from build123d import *

# Parameters (mm, degrees)
EXTRUDE_1_DEPTH = 30


with BuildPart() as part:
    # 草图1 → 拉伸-薄壁1 (new body)
    with BuildSketch(Plane(origin=(0, 0, 0), x_dir=(1, 0, 0), z_dir=(0, 1, 0))):
        Polygon((-10, -10), (70, -10), (70, 20), (49.5, 20), (49.5, 27), (26.5, 27), (26.5, 50), (20, 50), (20, 70), (-10, 70), align=None)
        Polygon((0, 0), (60, 0), (60, 10), (39.5, 10), (39.5, 17), (16.5, 17), (16.5, 40), (10, 40), (10, 60), (0, 60), align=None, mode=Mode.SUBTRACT)
    extrude(amount=EXTRUDE_1_DEPTH)


solid = part.part
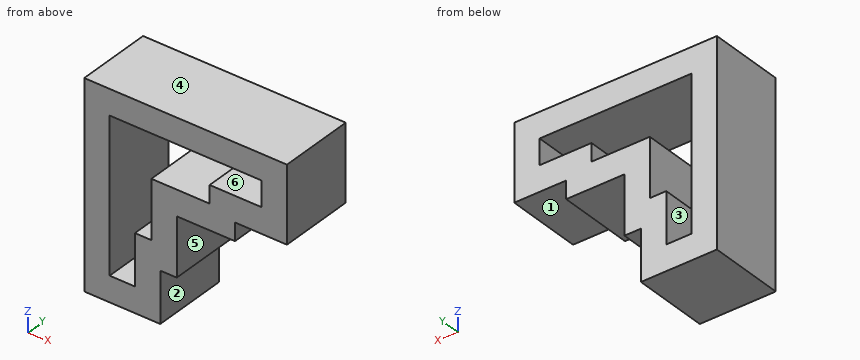
Input: part model. Units: mm. Frame: model coordinates. Face numbers are marked on the shaded views. A direction names the side the tool comes from. Give positions to 0.01 mm unless a question says otherwise; leave off trailing zeros. Order: outer loops, then holes, each group sorted by start corner. A loop starts at its lowest first (then second) coordinate and runs counter-clockwise, first axis right, second up.
Q1. Section A-A on x = 42. Output: boundary loops of the cut face in (y, z), and give its area (3 significant figures).
Checked values:
outline: (0, -27) - (30, -27) - (30, -10) - (0, -10) - close; (0, 0) - (30, 0) - (30, 10) - (0, 10) - close
area: 810 mm2
Q2. Contact query for flat-ended pins moving along their axis: pin 1 Ø10 at (y, z) = (19.5, -60) entering from +X; pin 2 Ø9 at (x, y) = (26.5, 16.5) entering from -Z; pin 3 Ø6 at (x, z) = (25, -24.5) entering from -Y; pin 4 Ø16.5 at (x, y) = (63, 22) entering from -Z. Output: stop coordinate, or through.
Checked values:
pin 1: stops at x = 20
pin 2: stops at z = -50
pin 3: stops at y = 0
pin 4: stops at z = -20
Q3. Set-up query: the marked faces 4, 5 and 6. Return all of +Z, -Z, +X, -X, +Y, -Y with unobstructed straight access to the full face (end or side cutting, diameter ignored); none if empty.
Checked values:
face 4: +Z, +X, -X, +Y, -Y
face 5: -Z, +X, +Y, -Y
face 6: +Y, -Y
Q4. Section C-C on z = -46. Output: boundary loops of the cut face in (x, y).
Checked values:
outline: (-10, 0) - (0, 0) - (0, 30) - (-10, 30) - close; (10, 0) - (26.5, 0) - (26.5, 30) - (10, 30) - close
Q5. Section B-B on y = 7.75. Output: boundary loops of the cut face in (x, z), and give its area (3 significant figures).
Checked values:
outline: (-10, -70) - (20, -70) - (20, -50) - (26.5, -50) - (26.5, -27) - (49.5, -27) - (49.5, -20) - (70, -20) - (70, 10) - (-10, 10) - close; hole (0, -60) - (10, -60) - (10, -40) - (16.5, -40) - (16.5, -17) - (39.5, -17) - (39.5, -10) - (60, -10) - (60, 0) - (0, 0) - close
area: 2,800 mm2
Q6. Ray query, probe 1 along Z at (x, y) = (35.5, 16.25); probe 2 along Z at (x, y) = (3, 2.25); probe 3 along X at (y, z) = (23.5, -42). Return the intervals inside material, ascending.
Checked values:
probe 1: z = -27 to -17, 0 to 10
probe 2: z = -70 to -60, 0 to 10
probe 3: x = -10 to 0, 10 to 26.5
Q7. Draft query along X for the marked faces 1, 2 and 3. Return one class per face: +X half, -X half, draft (parallel to the pull), parting line (faces both ways), or undercut.
Checked values:
face 1: draft
face 2: +X half
face 3: undercut
